Job drawing, mm, ordinate dimensions from the low corner. One solid piece. A direction names the side the tool comes from. Give positions to 0.01 mm unless a question says otherwise; leave off trailing zeros. Write each loop counter-clockwise with the first axis right and the second up, starting at its lowest first coordinate (ties: lowest second). Pieces come first, ordered by that corner, then holes. Notation, with made-up numbers: M 19,52.5 L 33,52.5 A25 cw 33,79.5 Z; hole C 54,-22.5 d1. An arc over 180 degrees is marked long. Use CSV: the item, a comma, the result in double quotes. Start each with the question number.
Item 1: Cut at C-C (x = 3). List the corners of the cut face in (y, z), then the cut area to 3 significant figures.
Item 2: Mould opens along X. For the marked faces 1, 2, 3 and 4 say: released by +X, released by -X, zero draft, split by the parting line, or undercut.
Item 3: Cut at D-D (z = 5). List the corners of the cut face in (x, y), then the cut area to 3 significant figures.
Item 4: Pin check, flat tips, straight feed: pin 1 (4 mm diameter, centred on x = 7.5, z = 6.5, fed in from -Y); pin 2 (2 mm diameter, centred on x = 2, z = 10, fed in from -Y); pin 3 (6 mm diameter, centred on x = 8.5, y = 13, fed in from +Z) (3 decimals). Stop position of each tip, or through.
Item 5: Which spindle directions (+Z, -Z, +X, -X, +Y, -Y) get a long thin tool onto all of the face, cutting with end or side? Do the marked faces 5 and 6. Say none if no direction does.
Item 6: Cut at A-A (z = 8). List the corners of the cut face in (x, y).
Item 7: Drill centre lines: line 1 (X direction, y = 2.75, z = 12); line 2 (Z direction, x = 6.25, y = 8); line 3 (Z direction, x = 5.75, y = 10). Where is each one in solid material? Low to high. Write a range as [from, to].
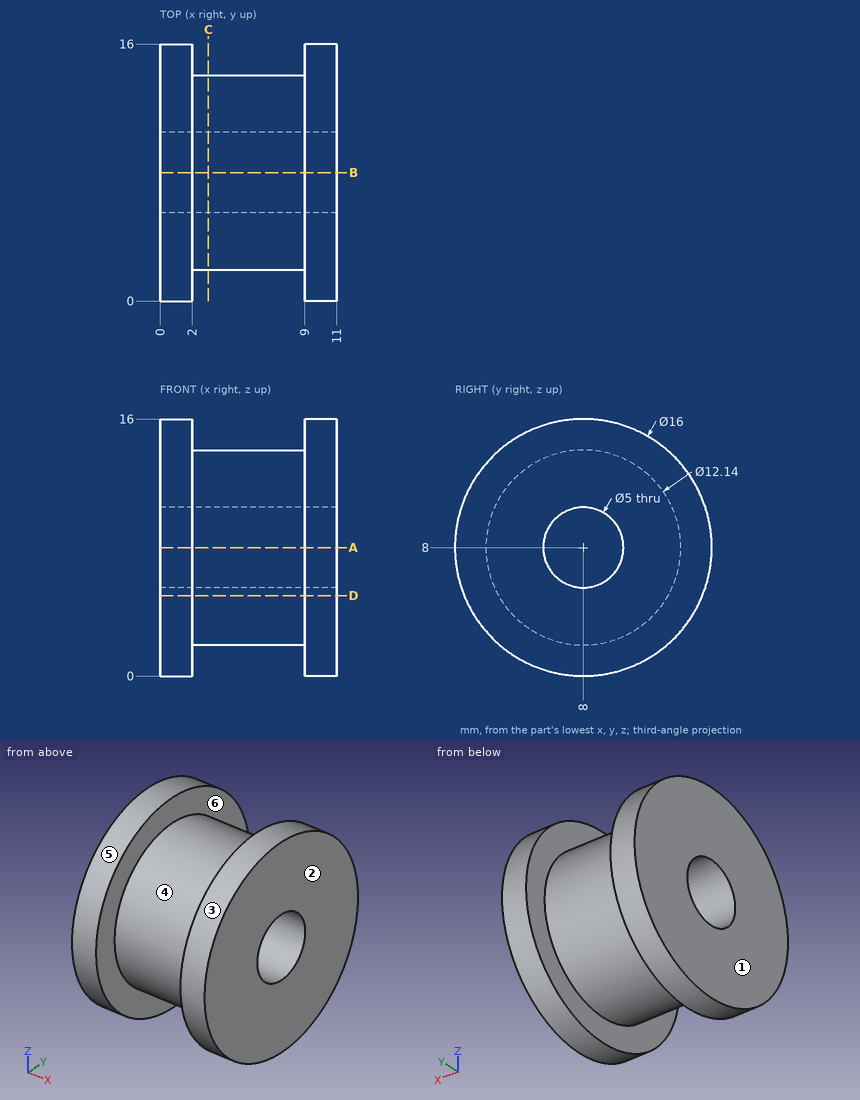
Worked answers:
1,outline,"C 8,8 d12.14; hole C 8,8 d5"
1,area,"96.1 mm^2"
2,face 1,"released by -X"
2,face 2,"released by +X"
2,face 3,"zero draft"
2,face 4,"undercut"
3,outline,"M 0,0.58 L 2,0.58 L 2,2.72 L 9,2.72 L 9,0.58 L 11,0.58 L 11,15.42 L 9,15.42 L 9,13.28 L 2,13.28 L 2,15.42 L 0,15.42 Z"
3,area,"133 mm^2"
4,pin 1,"stops at y = 0"
4,pin 2,"stops at y = 0.06"
4,pin 3,"stops at z = 15.735"
5,face 5,"+X, -X"
5,face 6,"none"
6,outline,"M 0,0 L 2,0 L 2,1.93 L 9,1.93 L 9,0 L 11,0 L 11,5.5 L 0,5.5 Z; M 0,10.5 L 11,10.5 L 11,16 L 9,16 L 9,14.07 L 2,14.07 L 2,16 L 0,16 Z"
7,line 1,"x = [0, 2], [9, 11]"
7,line 2,"z = [1.93, 5.5], [10.5, 14.07]"
7,line 3,"z = [2.27, 6.5], [9.5, 13.73]"
